Autodesk Inventor part; units mm, degrees
ref_plane "YZ Plane" through (0, 0, 0) normal (1, 0, 0) x (0, 1, 0)
ref_plane "XZ Plane" through (0, 0, 0) normal (0, 1, 0) x (-1, 0, 0)
ref_plane "XY Plane" through (0, 0, 0) normal (0, 0, 1) x (1, 0, 0)
sketch "Sketch1" plane through (0, 0, 0) normal (0, 1, 0) x (-1, 0, 0)
  line L0 (374, 0) -> (-374, 0)
  line L1 (-374, 0) -> (-374, 350)
  line L2 (-374, 350) -> (374, 350)
  line L3 (374, 350) -> (374, 0)
  point P0 (0, 0)
  point P1 (0, 0)
  dimension "d0" = 350
  dimension "d1" = 748
extrude "Extrusion1" add sketch "Sketch1" along normal blind 2012
shell "Shell1" thickness 15 removed faces 1 at (-124.6667, 670.6667, 350)
properties part number "PAX"
Input: part model. Units: mm. Frame: model coordinates. A direction names the side the tool comes from. Give positions to 0.01 mm unless a question says otherwise; leave off trailing zeros. Loops run counter-clockwise (first coordinate to the right, second up) from the corner with the lowest first, then second, coordinate; pieces in that order, holes last. Notation, with made-up numbers: M 68,-5 L 101,-5 A26 ccw 101,23 Z; hole C 2,85 d7. An arc over 180 degrees is marked long. Answer as CSV lines item,"result". Start each with the question number.
1. Section A-A on z = 177. Return loops of the section in (x, y).
2. Line query: L1, parallel to Y at x = -263, z = 52; L2, parallel to X at y = 308, z = 134; L3, parallel to Z at x = 24.5, y = 764. Output: solid intervals per line, ascending.
3. Pull-direction query (Y, two-part tool) for faces 1 (the face through (5, 2012, 177)), 2 (the face through (-374, 992, 177)), 3 (the face through (359, 992, 180)), 4 (the face through (5, 0, 177)); classes: released by +Y, released by -Y, zero draft, split by the parting line, or undercut.
4. Reachability of faces 5 (the face through (5, 15, 185)), 6 (the face through (362, 1001, 350)) from +Z, -Z, +X, -X, +Y, -Y: full face, straight path, thin tool, end or side. Return the list, or none.
5. Pin query (flat end, axial travel): P1, Ø4, axis at x = -153.5, y = 584.5, coming from the +Z side. Return the tip coordinate at first contact, or that it passes through.
6. Section B-B on y = 613. Return loops of the section in (x, z), plus the area to 3 significant figures.
7. Section C-C on x = 24. Return loops of the section in (y, z), plus the area to 3 significant figures.
Computed values:
1,outline,"M -374,0 L 374,0 L 374,2012 L -374,2012 Z; hole M -359,15 L 359,15 L 359,1997 L -359,1997 Z"
2,L1,"y = 0 to 15, 1997 to 2012"
2,L2,"x = -374 to -359, 359 to 374"
2,L3,"z = 0 to 15"
3,face 1,"released by +Y"
3,face 2,"zero draft"
3,face 3,"undercut"
3,face 4,"released by -Y"
4,face 5,"+Z"
4,face 6,"+Z, +X, -X, +Y, -Y"
5,P1,"stops at z = 15"
6,outline,"M -374,0 L 374,0 L 374,350 L 359,350 L 359,15 L -359,15 L -359,350 L -374,350 Z"
6,area,"21,300 mm²"
7,outline,"M 0,0 L 2012,0 L 2012,350 L 1997,350 L 1997,15 L 15,15 L 15,350 L 0,350 Z"
7,area,"40,200 mm²"
